```python
from build123d import *

# Parameters (mm, degrees)
SKETCH1_W                              = 215.5
SKETCH1_H                              = 25
BOSS_EXTRUDE1_DEPTH                    = 10
SKETCH2_W                              = 205.5
SKETCH2_H                              = 15
CUT_EXTRUDE1_DEPTH                     = 11
SKETCH3_W                              = 70
SKETCH3_H                              = 7
CUT_EXTRUDE2_DEPTH                     = 8.5
SKETCH4_W                              = 54.75
SKETCH4_H                              = 7
CUT_EXTRUDE3_DEPTH                     = 8.5
SKETCH5_W                              = 19.25
SKETCH5_H                              = 7
CUT_EXTRUDE4_DEPTH                     = 8.5
F_4_5_4_5_DIAMETER_HOLE1_D             = 4.5
F_4_5_4_5_DIAMETER_HOLE1_DEPTH         = 5
M4_CLEARANCE_HOLE1_D                   = 4.31
TAPPED_HOLE_FOR_1_4_20_HELICOIL1_D     = 6.7564
TAPPED_HOLE_FOR_1_4_20_HELICOIL1_DEPTH = 20.523
TAPPED_HOLE_FOR_1_4_20_HELICOIL1_TIP   = 2.029827343
F_4_5_4_5_DIAMETER_HOLE2_D             = 4.5
F_4_5_4_5_DIAMETER_HOLE2_DEPTH         = 215.5
FILLET1_R                              = 3


with BuildPart() as part:
    # Sketch1 → Boss-Extrude1 (new body)
    with BuildSketch(Plane(origin=(0, 5, 0), x_dir=(1, 0, 0), z_dir=(0, 1, 0))):
        with Locations((0, 10.5)):
            Rectangle(SKETCH1_W, SKETCH1_H)
    extrude(amount=-BOSS_EXTRUDE1_DEPTH)

    # Sketch2 → Cut-Extrude1 (cut, through all)
    with BuildSketch(Plane.XZ.offset(5)):
        with Locations((0, -15.5)):
            Rectangle(SKETCH2_W, SKETCH2_H)
    extrude(amount=-CUT_EXTRUDE1_DEPTH, mode=Mode.SUBTRACT)

    # Sketch3 → Cut-Extrude2 (cut)
    with BuildSketch(Plane(origin=(0, 0, -8), x_dir=(-1, 0, 0), z_dir=(0, 0, -1))):
        with Locations((-17.75, 0)):
            Rectangle(SKETCH3_W, SKETCH3_H)
    extrude(amount=-CUT_EXTRUDE2_DEPTH, mode=Mode.SUBTRACT)

    # Sketch4 → Cut-Extrude3 (cut)
    with BuildSketch(Plane(origin=(0, 0, -8), x_dir=(-1, 0, 0), z_dir=(0, 0, -1))):
        with Locations((54.625, 0)):
            Rectangle(SKETCH4_W, SKETCH4_H)
    extrude(amount=-CUT_EXTRUDE3_DEPTH, mode=Mode.SUBTRACT)

    # Sketch5 → Cut-Extrude4 (cut)
    with BuildSketch(Plane(origin=(0, 0, -8), x_dir=(-1, 0, 0), z_dir=(0, 0, -1))):
        with Locations((-72.375, 0)):
            Rectangle(SKETCH5_W, SKETCH5_H)
    extrude(amount=-CUT_EXTRUDE4_DEPTH, mode=Mode.SUBTRACT)

    # Ø4.5 (4.5) Diameter Hole1
    with Locations(Plane(origin=(-102.75, 0, 0), x_dir=(0, 0, -1), z_dir=(1, 0, 0))):
        with Locations((17, 0)):
            Hole(F_4_5_4_5_DIAMETER_HOLE1_D / 2, depth=F_4_5_4_5_DIAMETER_HOLE1_DEPTH)

    # M4 Clearance Hole1 (through all)
    with Locations(Plane.XY.offset(2)):
        with Locations((-99.75154, 0), (92.2496, 0)):
            Hole(M4_CLEARANCE_HOLE1_D / 2)

    # Tapped Hole for 1/4-20 Helicoil1
    with Locations(Plane.XY.offset(2)):
        with Locations((57.75, 0), (-22.25, 0)):
            Hole(TAPPED_HOLE_FOR_1_4_20_HELICOIL1_D / 2, depth=TAPPED_HOLE_FOR_1_4_20_HELICOIL1_DEPTH)
            with Locations((0, 0, -(TAPPED_HOLE_FOR_1_4_20_HELICOIL1_DEPTH + TAPPED_HOLE_FOR_1_4_20_HELICOIL1_TIP / 2))):  # 118° drill point
                Cone(0, TAPPED_HOLE_FOR_1_4_20_HELICOIL1_D / 2, TAPPED_HOLE_FOR_1_4_20_HELICOIL1_TIP, mode=Mode.SUBTRACT)

    # Ø4.5 (4.5) Diameter Hole2
    with Locations(Plane(origin=(107.75, 0, 0), x_dir=(0, 0, -1), z_dir=(1, 0, 0))):
        with Locations((17, 0)):
            Hole(F_4_5_4_5_DIAMETER_HOLE2_D / 2, depth=F_4_5_4_5_DIAMETER_HOLE2_DEPTH)

    # Fillet1
    fillet1_edges = [part.edges().sort_by_distance(p)[0] for p in [
        (-17.25, 3.5, -3.75),
        (-17.25, -3.5, -3.75),
        (52.75, -3.5, -3.75),
        (52.75, 3.5, -3.75),
        (-82, 3.5, -3.75),
        (-82, -3.5, -3.75),
        (-27.25, -3.5, -3.75),
        (-27.25, 3.5, -3.75),
        (62.75, -3.5, -3.75),
        (82, -3.5, -3.75),
        (82, 3.5, -3.75),
        (62.75, 3.5, -3.75),
    ]]
    fillet(fillet1_edges, radius=FILLET1_R)


solid = part.part
```
Design review of the part built by this model. Coordinates are the model's own, in mm. A direction names the side the tool comes from. Coordinates: 2 decimals unless noted, no trailing zeros. Loops run counter-clockwise (first coordinate to the right, second up) from the corner with the lowest first, then second, coordinate; pieces in that order, holes last. Notation, with made-up numbers: (59, 14) -> (102, 14) arc R26 cw to (102, 47) -> close; hole circle Ø3 at (39, 57.5). An arc over 180 degrees is marked (long way). Answer as a JSON object with one key per item and string values.
Q1. Take a section at A-A on z = -2.5. Give the number of separate pieces and of enclosed holes in the cut face, plus the area to 3 significant figures.
Answer block:
{"separate pieces": "1", "enclosed holes": "7", "area": "1,070 mm^2"}
Q2. Take a section at B-B on x = -22.25. Give the boundary of the cut face in (y, z), plus the area to 3 significant figures.
Answer block:
{"outline": "(-5, -8) -> (-3.38, -8) -> (-3.38, 2) -> (-5, 2) -> close; (3.38, -8) -> (5, -8) -> (5, 2) -> (3.38, 2) -> close", "area": "32.4 mm^2"}
Q3. Take a section at C-C on x = -0.5. Give the boundary of the cut face in (y, z).
Answer block:
{"outline": "(-5, -8) -> (-3.5, -8) -> (-3.5, 0.5) -> (3.5, 0.5) -> (3.5, -8) -> (5, -8) -> (5, 2) -> (-5, 2) -> close"}
Q4. The part is to be moulded in two halves that separate along Y. For faces 1 (the flat face through (105, 0, -23)), 2 (the flat face through (-2, -5, -2)), 3 (the flat face through (-54, -3.5, -4)), say which applies: +Y half, -Y half, draft (parallel to the pull), parting line (faces both ways), or undercut.
Answer block:
{"face 1": "draft", "face 2": "-Y half", "face 3": "undercut"}
Q5. Tool access review of faces 4 (the flat face through (107.75, 0, -10)), 5 (the flat face through (18, 3.5, -4)), 6 (the flat face through (102.75, 0, -14)): name each direction out of +Z, -Z, +X, -X, +Y, -Y from which nothing blocks a thin tool from reaching the whole face with its end or side.
Answer block:
{"face 4": "+Z, -Z, +X, +Y, -Y", "face 5": "-Z", "face 6": "-Z, +Y, -Y"}
Q6. To check wall thickness, follow L1, parallel to Y at x = 19.5, z = -6; L2, parallel to X at y = -0.5, z = -9; L3, parallel to X at y = 2.5, z = -4. State the ranges of each line that lie inside material, in increasing order.
Answer block:
{"L1": "y = -5 to -3.5, 3.5 to 5", "L2": "x = -107.75 to -102.75, 102.75 to 107.75", "L3": "x = -107.75 to -81.24, -28.01 to -24.52, -19.98 to -16.49, 51.99 to 55.48, 60.02 to 63.51, 81.24 to 107.75"}
Q7. Clearance check with flat-ended pins moving along their axes: pin 1 Ø3.5 at (x, y) = (92.25, 0) entering from +Z; pin 2 Ø5.5 at (x, y) = (-47.5, -0.5) entering from -Z; pin 3 Ø5 at (x, y) = (74.5, 4) entering from -Z. State where each tip first meets the part, or that it passes through.
Answer block:
{"pin 1": "passes through", "pin 2": "stops at z = 0.5", "pin 3": "stops at z = -8"}
